Could you check a few things on this model? Use its own coordinates, in mm. A direction names the side the tool comes from. Give positions to 0.01 mm unless a question says otherwise; leave off trailing zeros. Loops run counter-clockwise (first coordinate to the right, second up) from the corner with the lowest first, then second, coordinate; pieces in that order, holes last. Notation, with made-up numbers: (40.5, 59) -> (57.5, 59) arc R15 cw to (57.5, 68) -> close; hole circle Ø11 at (-4, -14). An arc over 180 degrees is marked (long way). Put each result on its own line as item: value.
```python
from build123d import *

# Parameters (mm, degrees)
F2_DEPTH  = 15
F3_SIZE2  = 10
F3_SIZE   = 5
F4_W      = 78.75
F4_H      = 51.75
F4_R      = 5
F4_R_2    = 3.75
F4_R_3    = 1
F5_DEPTH  = 15.001
F6_W      = 96
F6_H      = 90
F7_DEPTH  = 8
F8_R      = 1.425
F9_DEPTH  = 1.5
F10_W     = 8.4
F10_H     = 51.75
F11_DEPTH = 4
F12_R     = 7
F13_DEPTH = 5
F15_DEPTH = 5


with BuildPart() as f2:
    # F1 (on Top) → F2 (new body)
    with BuildSketch(Plane.XY):
        with BuildLine():
            Line((45.5, 52.5), (-45.5, 52.5))
            ThreePointArc((-45.5, 52.5), (-52.5710678119, 49.5710678119), (-55.5, 42.5))
            Line((-55.5, 42.5), (-55.5, -42.5))
            ThreePointArc((-55.5, -42.5), (-52.5710678119, -49.5710678119), (-45.5, -52.5))
            Line((-45.5, -52.5), (45.5, -52.5))
            ThreePointArc((45.5, -52.5), (52.5710678119, -49.5710678119), (55.5, -42.5))
            Line((55.5, -42.5), (55.5, 42.5))
            ThreePointArc((55.5, 42.5), (52.5710678119, 49.5710678119), (45.5, 52.5))
        make_face()
    extrude(amount=-F2_DEPTH)

    # F3
    f3_edges = [f2.edges().sort_by_distance(p)[0] for p in [
        (-55.5, 0, 0),
    ]]
    f3_side = f2.faces().sort_by_distance((0, 0, 0))[0]
    chamfer(f3_edges, length=F3_SIZE, length2=F3_SIZE2, reference=f3_side)

    # F4 (on Top) → F5 (cut, through all)
    with BuildSketch(Plane.XY):
        with Locations((-0.225, 8.875)):
            Rectangle(F4_W, F4_H)
        with Locations((4.65, -34.75)):
            Circle(F4_R)
        with Locations((37.15, -34.75)):
            Circle(F4_R_2)
        with Locations((16.9, -34.75)):
            Circle(F4_R_3)
        with Locations((19.65, -32)):
            Circle(F4_R_3)
        with Locations((22.4, -34.75)):
            Circle(F4_R_3)
        with Locations((19.65, -37.5)):
            Circle(F4_R_3)
    extrude(amount=-F5_DEPTH, mode=Mode.SUBTRACT)

    # F6 (on face) → F7 (cut)
    with BuildSketch(Plane(origin=(0, 0, -15), x_dir=(1, 0, 0), z_dir=(0, 0, -1))):
        Rectangle(F6_W, F6_H)
    extrude(amount=-F7_DEPTH, mode=Mode.SUBTRACT)

    # F8 (on face) → F9 (join)
    with BuildSketch(Plane(origin=(0, 0, -7), x_dir=(1, 0, 0), z_dir=(0, 0, -1))):
        with Locations((43.9, -40.9)):
            Circle(F8_R)
        with Locations((-43.9, -40.9)):
            Circle(F8_R)
        with Locations((-43.9, 24.9)):
            Circle(F8_R)
        with Locations((43.9, 24.9)):
            Circle(F8_R)
    extrude(amount=F9_DEPTH)

    # F10 (on face) → F11 (cut)
    with BuildSketch(Plane(origin=(0, 0, -7), x_dir=(1, 0, 0), z_dir=(0, 0, -1))):
        with Locations((-43.8, -8.875)):
            Rectangle(F10_W, F10_H)
    extrude(amount=-F11_DEPTH, mode=Mode.SUBTRACT)

    # F12 (on face) → F13 (cut)
    with BuildSketch(Plane(origin=(0, 0, -7), x_dir=(1, 0, 0), z_dir=(0, 0, -1))):
        with Locations((4.65, 34.75)):
            Circle(F12_R)
        with Locations((19.65, 34.75)):
            Circle(F12_R)
    extrude(amount=-F13_DEPTH, mode=Mode.SUBTRACT)

    # F14 (on face) → F15 (cut)
    with BuildSketch(Plane(origin=(0, 0, -7), x_dir=(1, 0, 0), z_dir=(0, 0, -1))):
        with BuildLine():
            Line((-38.6, 22), (29.15, 22))
            Line((29.15, 22), (29.15, 26))
            Line((29.15, 26), (-17.4708836394, 26))
            ThreePointArc((-17.4708836394, 26), (-26.4833749709, 28.2735239814), (-33.3390120735, 34.55))
            ThreePointArc((-33.3390120735, 34.55), (-43.1741435319, 34.8175816996), (-40.0375, 25.4921928002))
            ThreePointArc((-40.0375, 25.4921928002), (-38.9992189406, 24.7718816144), (-38.6, 23.5729237336))
            Line((-38.6, 23.5729237336), (-38.6, 22))
        make_face()
    extrude(amount=-F15_DEPTH, mode=Mode.SUBTRACT)


solid = f2.part
```
1. I'm going to push flat-ended pins straight in: pin 1 (0.9 mm diameter, centred on x = -44.5, y = 40.5, fed in from -Z); pin 2 (7 mm diameter, centred on x = 4, y = -37, fed in from -Z); pin 3 (3 mm diameter, centred on y = -6, z = -5, fed in from -X); pin 4 (8.5 mm diameter, centred on x = 37.15, y = -34.75, fed in from +Z). Where does each tip first touch, or does it pass through?
Recorded:
pin 1: stops at z = -8.5
pin 2: stops at z = -2
pin 3: stops at x = -53.75
pin 4: stops at z = 0
2. I need wall thicknesses on line 1 (Y direction, x = 30, z = -12.5); line 2 (X direction, y = 14, z = -10); line 3 (X direction, y = -23.5, z = -4). Which ranges of each line are inside material? Lowest first, please.
Recorded:
line 1: y = -52.5 to -45, 45 to 52.5
line 2: x = -55.5 to -48, 48 to 55.5
line 3: x = -52.5 to -38.6, 29.15 to 52.5
3. If we section it at A-A (y = 17): List the corners of the cut face in (x, z) for me.
Recorded:
outline: (-55.5, -15) -> (-48, -15) -> (-48, -3) -> (-39.6, -3) -> (-39.6, 0) -> (-50.5, 0) -> (-55.5, -10) -> close; (39.15, -7) -> (48, -7) -> (48, -15) -> (55.5, -15) -> (55.5, -10) -> (50.5, 0) -> (39.15, 0) -> close
4. If we section it at D-D (y = 40.9): List the corners of the cut face in (x, z) for me (3 decimals), then the cut area to 3 significant figures.
Recorded:
outline: (-55.5, -15) -> (-48, -15) -> (-48, -7) -> (-45.325, -7) -> (-45.325, -8.5) -> (-42.475, -8.5) -> (-42.475, -7) -> (42.475, -7) -> (42.475, -8.5) -> (45.325, -8.5) -> (45.325, -7) -> (48, -7) -> (48, -15) -> (55.5, -15) -> (55.5, -10) -> (50.5, 0) -> (-50.5, 0) -> (-55.5, -10) -> close
area: 856 mm^2
5. If we section it at C-C (x = -10): List the corners of the cut face in (y, z) for me.
Recorded:
outline: (-52.5, -15) -> (-45, -15) -> (-45, -7) -> (-26, -7) -> (-26, -2) -> (-22, -2) -> (-22, -7) -> (-17, -7) -> (-17, 0) -> (-47.5, 0) -> (-52.5, -10) -> close; (34.75, -7) -> (45, -7) -> (45, -15) -> (52.5, -15) -> (52.5, -10) -> (47.5, 0) -> (34.75, 0) -> close
6. Thinking about a two-plate mould opening in Y: for faces 4 (the face through (-55.5, 1, -12)), 5 (the face through (-43.242, 42.164, -7.74)), 6 (the face through (50.769, -47.886, -5.07)), 7 (the face through (-5, 34.75, -3)), which applies, pulls with the +Y half, pulls with the -Y half, needs draft (parallel to the pull), parting line crosses it, or undercut?
Recorded:
face 4: needs draft
face 5: undercut
face 6: pulls with the -Y half
face 7: undercut
7. If we section it at B-B (x = 37.15): List the corners of the cut face in (y, z) for me, then the cut area to 3 significant figures.
Recorded:
outline: (-52.5, -15) -> (-45, -15) -> (-45, -7) -> (-38.5, -7) -> (-38.5, 0) -> (-47.5, 0) -> (-52.5, -10) -> close; (-31, -7) -> (-17, -7) -> (-17, 0) -> (-31, 0) -> close; (34.75, -7) -> (45, -7) -> (45, -15) -> (52.5, -15) -> (52.5, -10) -> (47.5, 0) -> (34.75, 0) -> close
area: 390 mm^2
8. For faces 1 (the face through (1, 52.5, -12)), 2 (the face through (39.15, 9, -3)), 3 (the face through (-48, 1, -10)), which set-ups out of +Z, -Z, +X, -X, +Y, -Y let a thin tool reach every point of the face, with its end or its side?
Recorded:
face 1: +Z, -Z, +X, -X, +Y
face 2: +Z, -Z
face 3: -Z
